Can you work these out from the model? Positions are in its coordinate system, mm. Face numbers are marked on the shaded views. A direction names the side the tool comes from. Round coordinates to 2 decimals unless told otherwise and drop trailing zeros. Order: outer loops, then holes, each group sorted by start corner. A loop starts at its lowest first (then second) coordinate and runs counter-clockwise, first axis right, second up. Notation, with made-up numbers: M 8.5,70.5 L 18.5,70.5 A14 cw 18.5,79.5 Z; hole C 83.25,82.25 d4. An arc over 180 degrees is marked long. One line per question, with ' | ' between items.
```python
from build123d import *

# Parameters (mm, degrees)
SKETCH_2_W          = 40
SKETCH_2_H          = 40
FILLET_1_RADIUS     = 20
FILLET_1_LENGTH     = 40
SKETCH_3_R          = 6
CUT_EXTRUDE_1_DEPTH = 477.759897642
SKETCH_4_R          = 10
CUT_EXTRUDE_2_DEPTH = 10
SKETCH_5_R          = 15
CUT_EXTRUDE_3_DEPTH = 477.759897642


with BuildPart() as part:
    # 扫描1: sweep along a path in 草图1
    with BuildLine(Plane(origin=(0, 0, 0), x_dir=(1, 0, 0), z_dir=(0, 1, 0))) as sweep_1_path:
        Line((0, 0), (0, -30.887892176))
        ThreePointArc((0, -30.887892176), (-4.698256626, -47.006880426), (-17.321452148, -58.077125787))
        Line((-17.321452148, -58.077125787), (-242.678547852, -163.162865333))
        ThreePointArc((-242.678547852, -163.162865333), (-255.301743374, -174.233110694), (-260, -190.352098945))
        Line((-260, -190.352098945), (-260, -370))
    # 草图2 → 扫描1 (sweep)
    with BuildSketch(Plane.XY):
        Rectangle(SKETCH_2_W, SKETCH_2_H)
    sweep(path=sweep_1_path.line)

    # 圆角1: full round fillet: the end face becomes a half cylinder, R = half its width
    fillet_1_face = Plane((-260, 0, 370), x_dir=(1, 0, 0), z_dir=(0, 0, 1))  # on the end face: x along it, z out of the body
    fillet_1_slab = fillet_1_face.offset(-FILLET_1_RADIUS / 2) * Box(FILLET_1_LENGTH, 2 * FILLET_1_RADIUS, FILLET_1_RADIUS, mode=Mode.PRIVATE)  # the body's end, R deep
    fillet_1_round = Plane((-260, 0, 350), x_dir=(0, 0, 1), z_dir=(1, 0, 0)) * Cylinder(FILLET_1_RADIUS, FILLET_1_LENGTH, mode=Mode.PRIVATE)  # its axis R under the face
    add(fillet_1_slab - fillet_1_round, mode=Mode.SUBTRACT)

    # 草图3 → 切除-拉伸1 (cut, through all)
    with BuildSketch(Plane.ZY.offset(280)):
        with Locations((350, 0)):
            Circle(SKETCH_3_R)
    extrude(amount=-CUT_EXTRUDE_1_DEPTH, mode=Mode.SUBTRACT)

    # 草图4 → 切除-拉伸2 (cut)
    with BuildSketch(Plane(origin=(0, 0, 0), x_dir=(-1, 0, 0), z_dir=(0, 0, -1))):
        Circle(SKETCH_4_R)
    extrude(amount=-CUT_EXTRUDE_2_DEPTH, mode=Mode.SUBTRACT)

    # 草图5 → 切除-拉伸3 (cut, through all)
    with BuildSketch(Plane.ZY.offset(280)):
        with Locations((207.352098945, 0)):
            Circle(SKETCH_5_R)
    extrude(amount=-CUT_EXTRUDE_3_DEPTH, mode=Mode.SUBTRACT)


solid = part.part
```
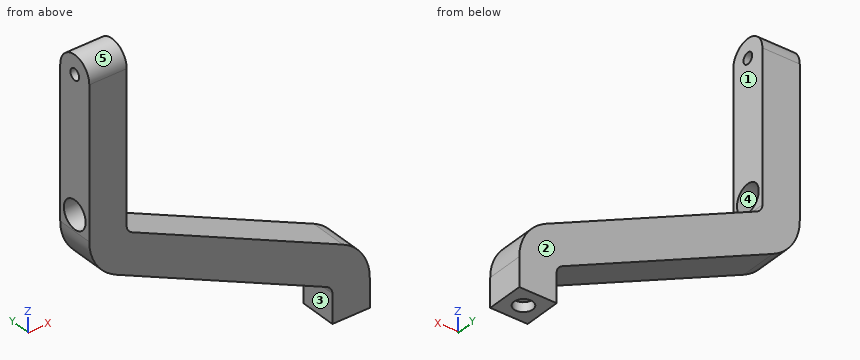
(1) Will these pins go through, and if not, where does the flat tip stop? pin 1 Ø6 at (x, y) = (-70, -10.5) entering from +Z; pin 2 Ø6 at (y, z) = (2, 153.5) entering from -X; pin 3 Ø6 at (x, y) = (0, -4.5) entering from -Z.
Final values:
pin 1: z = 106.11 | pin 2: x = -266.8 | pin 3: z = 10
(2) Thinking about a two-plate mould opening in Z: for the marked faces 3, 4 and 5, which applies, released by +Z, released by -Z, zero draft, split by the parting line, or undercut?
Final values:
face 3: zero draft | face 4: undercut | face 5: released by +Z
(3) If we section it at B-B on z = 338.5: Please give me the cut outline in (x, y).
Final values:
outline: M -280,-20 L -240,-20 L -240,20 L -280,20 Z
(4) If we section it at D-D on z = 123: Please give me the cut outline in (x, y), plus the area to 3 significant figures.
Final values:
outline: M -203.87,-20 L -109.22,-20 L -109.22,20 L -203.87,20 Z | area: 3,790 mm^2
(5) If we section it at A-A on y = 0: Please give me the cut outline in (x, z), plus the area to 3 significant figures.
Final values:
outline: M -280,190.35 A50 ccw -251.13,145.04 L -25.77,39.95 A10 cw -20,30.89 L -20,0 L -10,0 L -10,10 L 10,10 L 10,0 L 20,0 L 20,30.89 A50 ccw -8.87,76.2 L -234.23,181.29 A10 cw -240,190.35 L -240,192.35 L -280,192.35 Z; M -280,222.35 L -240,222.35 L -240,344 L -280,344 Z; M -280,356 L -240,356 L -240,370 L -280,370 Z | area: 19,200 mm^2
(6) If we section it at C-C on x = 0: Please give me the cut outline in (y, z), plus the area to 3 significant figures.
Final values:
outline: M -20,0 L -10,0 L -10,10 L 10,10 L 10,0 L 20,0 L 20,70.89 L -20,70.89 Z | area: 2,640 mm^2
(7) Please list where these lines run through material, in increasing order: probe 1 along Y at (x, z) = (0, 4.25); probe 2 along Y at (x, z) = (-269, 350); probe 3 along Z at (x, y) = (-262, 2.5). Write a range as [from, to].
Final values:
probe 1: [-20, -10], [10, 20] | probe 2: [-20, -6], [6, 20] | probe 3: [151.93, 192.56], [222.14, 344.55], [355.45, 369.84]
(8) On a 3-axis mill with a long thin cutter (end or side, diameter ignored), from which of +Z, -Z, +X, -X, +Y, -Y can I reach the whole of each face in a straight line? I mean the marked faces 1 and 2. Say none if no direction works.
Final values:
face 1: +Z, +X, +Y, -Y | face 2: +Z, -Z, +X, -X, +Y
